Part model, mm, in its own coordinate system. Round coordinates to 2 decimals unless told otherwise and drop trailing zeros. Loops run counter-clockwise (first coordinate to the right, second up) from the corner with the lowest first, then second, coordinate; pieces in that order, holes last. Notation, with made-up numbers: (49.5, -38) - (87.5, -38) arc R22 ccw to (87.5, -24) - close; hole circle Ø10 at (-6, 19.5). An arc over 180 degrees is marked (long way). Put each result on its own line as item: value.
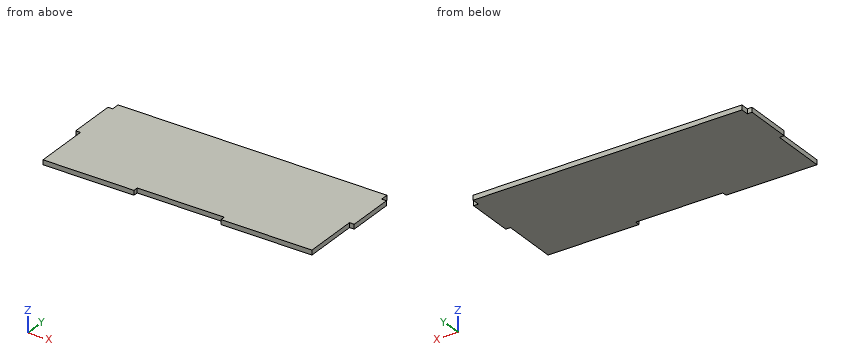
from build123d import *

# Parameters (mm, degrees)
F0_W     = 3
F0_H     = 30
F1_DEPTH = 3


with BuildPart() as f1:
    # F0 (on Top) → F1 (new body)
    with BuildSketch(Plane.XY):
        with Locations((86.5, 15)):
            Rectangle(F0_W, F0_H)
        with Locations((-86.5, 15)):
            Rectangle(F0_W, F0_H)
        Polygon((85, 30), (85, 35), (-85, 35), (-85, 30), (-85, 0), (-85, -35), (-27.5, -35), (-27.5, -32), (27.5, -32), (27.5, -35), (85, -35), (85, 0), align=None)
    extrude(amount=F1_DEPTH)


solid = f1.part
1. Pin check, flat tips, straight feed: P1, Ø0.9, axis at x = -87, z = 1, coming from the -Y side; P2, Ø0.9, axis at x = -86, z = 2, coming from the +Y side; P3, Ø1.5, axis at y = -13, z = 2, coming from the +X side. Stop position of each tip, or through.
A:
P1: stops at y = 0
P2: stops at y = 30
P3: stops at x = 85
2. Band-saw the part on A-A (z = 2.5). List the corners of the cut face in (x, y), plus the area to 3 significant figures.
A:
outline: (-88, 0) - (-85, 0) - (-85, -35) - (-27.5, -35) - (-27.5, -32) - (27.5, -32) - (27.5, -35) - (85, -35) - (85, 0) - (88, 0) - (88, 30) - (85, 30) - (85, 35) - (-85, 35) - (-85, 30) - (-88, 30) - close
area: 11,900 mm²
3. Band-saw the part on C-C (x = 19). List the corners of the cut face in (y, z), plus the area to 3 significant figures.
A:
outline: (-32, 0) - (35, 0) - (35, 3) - (-32, 3) - close
area: 201 mm²
4. Band-saw the part on B-B (y = -3). List the corners of the cut face in (x, z).
A:
outline: (-85, 0) - (85, 0) - (85, 3) - (-85, 3) - close
5. Probe line 1 along Y through (x, z) = (2, 2.6); line 2 along X through (y, z) = (-17.5, 2.95). List the from-to ranges inside material, lowest first. Write a range as [from, to].
A:
line 1: y = [-32, 35]
line 2: x = [-85, 85]
